CAD build for the part. Positions are in the model's coordinates, mm. Face numbers are marked on the shaded views. Give positions to 0.01 mm unless a question says otherwise; leave off trailing zeros. Loops run counter-clockwise (first coordinate to the right, second up) from the corner with the lowest first, then second, coordinate; pieces in that order, holes last.
```python
from build123d import *

# Parameters (mm, degrees)
BASPROSKE_W         = 8
BASPROSKE_H         = 8.5
TOOTHCUT_DEPTH      = 15.439529078
TEETHCUTS_COUNT     = 15
TEETHCUTS_ANGLE     = 336
BORSKE_R            = 0.75
BORE_DEPTH          = 50.0000508
SKETCH1_R           = 2.8
CUT_EXTRUDE2_DEPTH  = 1
BOSS_EXTRUDE2_START = 1.6
SKETCH2_R           = 0.75
BOSS_EXTRUDE2_DEPTH = 1.6


with BuildPart() as part:
    # BasProSke → Base-Revolve (revolve)
    with BuildSketch(Plane(origin=(0, 0, 0), x_dir=(1, 0, 0), z_dir=(0, 1, 0)), mode=Mode.PRIVATE) as base_revolve_sk:
        with Locations((4, 4.25)):
            Rectangle(BASPROSKE_W, BASPROSKE_H)
    revolve(base_revolve_sk.sketch.rotate(Axis((-10, 0, 0), (1, 0, 0)), 180), axis=Axis((-10, 0, 0), (1, 0, 0)))

    # TooCutSke → ToothCut (cut, through all)
    with BuildSketch(Plane(origin=(0, 0, 0), x_dir=(0, 0, -1), z_dir=(1, 0, 0))):
        with BuildLine():
            ThreePointArc((0.619547138, 6.21821215), (0, 6.249), (-0.619547138, 6.21821215))
            ThreePointArc((-0.619547138, 6.21821215), (-0.827197364, 7.394441061), (-1.477319646, 8.396426134))
            ThreePointArc((-1.477319646, 8.396426134), (0, 8.5254), (1.477319646, 8.396426134))
            ThreePointArc((1.477319646, 8.396426134), (0.827197364, 7.394441061), (0.619547138, 6.21821215))
        make_face()
    toothcut = extrude(amount=TOOTHCUT_DEPTH, mode=Mode.SUBTRACT)

    # TeethCuts: ToothCut ×15 about axis
    teethcuts_axis = Axis((-10, 0, 0), (1, 0, 0))
    for i in range(1, TEETHCUTS_COUNT):
        add(toothcut.rotate(teethcuts_axis, i * TEETHCUTS_ANGLE / (TEETHCUTS_COUNT - 1)), mode=Mode.SUBTRACT)

    # BorSke → Bore (cut, symmetric)
    with BuildSketch(Plane(origin=(0, 0, 0), x_dir=(0, 0, -1), z_dir=(1, 0, 0))):
        with Locations(Location((0, 0, 0), (0, 0, 180))):
            Circle(BORSKE_R)
    extrude(amount=BORE_DEPTH, both=True, mode=Mode.SUBTRACT)

    # Sketch1 → Cut-Extrude2 (cut)
    with BuildSketch(Plane(origin=(8, 0, 0), x_dir=(0, 0, -1), z_dir=(1, 0, 0))):
        Circle(SKETCH1_R)
    extrude(amount=-CUT_EXTRUDE2_DEPTH, mode=Mode.SUBTRACT)

    # Sketch2 → Boss-Extrude2 (add)
    with BuildSketch(Plane.ZY.offset(BOSS_EXTRUDE2_START)):
        with BuildLine():
            ThreePointArc((6.248908444, -0.033826967), (7.425583576, 0.045669992), (8.480693328, 0.572573726))
            ThreePointArc((8.480693328, 0.572573726), (8.453436111, 0.888491938), (8.414414603, 1.203173673))
            ThreePointArc((8.414414603, 1.203173673), (7.272812084, 1.499193643), (6.105321779, 1.332308887))
            ThreePointArc((6.105321779, 1.332308887), (5.94315217, 1.931047198), (5.722420591, 2.510757571))
            ThreePointArc((5.722420591, 2.510757571), (6.765032487, 3.061978551), (7.514612153, 3.972480862))
            ThreePointArc((7.514612153, 3.972480862), (7.361215932, 4.25), (7.197575419, 4.521604593))
            ThreePointArc((7.197575419, 4.521604593), (6.034267454, 4.327700716), (5.035590135, 3.700382817))
            ThreePointArc((5.035590135, 3.700382817), (4.643912014, 4.181397159), (4.206474231, 4.621209316))
            ThreePointArc((4.206474231, 4.621209316), (4.934745822, 5.5488432), (5.249186267, 6.685509968))
            ThreePointArc((5.249186267, 6.685509968), (4.996174644, 6.876644452), (4.736210056, 7.058209001))
            ThreePointArc((4.736210056, 7.058209001), (3.752343161, 6.407909019), (3.095159209, 5.428626941))
            ThreePointArc((3.095159209, 5.428626941), (2.541697283, 5.708745565), (1.963190262, 5.932611987))
            ThreePointArc((1.963190262, 5.932611987), (2.251196774, 7.076262451), (2.076128389, 8.242553664))
            ThreePointArc((2.076128389, 8.242553664), (1.767249372, 8.314254606), (1.455910948, 8.374384951))
            ThreePointArc((1.455910948, 8.374384951), (0.821604647, 7.380131638), (0.619547138, 6.21821215))
            ThreePointArc((0.619547138, 6.21821215), (0, 6.249), (-0.619547138, 6.21821215))
            ThreePointArc((-0.619547138, 6.21821215), (-0.821604647, 7.380131638), (-1.455910948, 8.374384951))
            ThreePointArc((-1.455910948, 8.374384951), (-1.767249372, 8.314254606), (-2.076128389, 8.242553664))
            ThreePointArc((-2.076128389, 8.242553664), (-2.251196774, 7.076262451), (-1.963190262, 5.932611987))
            ThreePointArc((-1.963190262, 5.932611987), (-2.541697283, 5.708745565), (-3.095159209, 5.428626941))
            ThreePointArc((-3.095159209, 5.428626941), (-3.752343161, 6.407909019), (-4.736210056, 7.058209001))
            ThreePointArc((-4.736210056, 7.058209001), (-4.996174644, 6.876644452), (-5.249186267, 6.685509968))
            ThreePointArc((-5.249186267, 6.685509968), (-4.934745822, 5.5488432), (-4.206474231, 4.621209316))
            ThreePointArc((-4.206474231, 4.621209316), (-4.643912014, 4.181397159), (-5.035590135, 3.700382817))
            ThreePointArc((-5.035590135, 3.700382817), (-6.034267454, 4.327700716), (-7.197575419, 4.521604593))
            ThreePointArc((-7.197575419, 4.521604593), (-7.361215932, 4.25), (-7.514612153, 3.972480862))
            ThreePointArc((-7.514612153, 3.972480862), (-6.765032487, 3.061978551), (-5.722420591, 2.510757571))
            ThreePointArc((-5.722420591, 2.510757571), (-5.94315217, 1.931047198), (-6.105321779, 1.332308887))
            ThreePointArc((-6.105321779, 1.332308887), (-7.272812084, 1.499193643), (-8.414414603, 1.203173673))
            ThreePointArc((-8.414414603, 1.203173673), (-8.453436111, 0.888491938), (-8.480693328, 0.572573726))
            ThreePointArc((-8.480693328, 0.572573726), (-7.425583576, 0.045669992), (-6.248908444, -0.033826967))
            ThreePointArc((-6.248908444, -0.033826967), (-6.214767324, -0.653198367), (-6.119387823, -1.266133354))
            ThreePointArc((-6.119387823, -1.266133354), (-7.253821434, -1.58853763), (-8.17632506, -2.323296905))
            ThreePointArc((-8.17632506, -2.323296905), (-8.083980389, -2.626644452), (-7.980385583, -2.926336609))
            ThreePointArc((-7.980385583, -2.926336609), (-6.802183806, -2.978535323), (-5.694903257, -2.572562515))
            ThreePointArc((-5.694903257, -2.572562515), (-5.411792748, -3.1245), (-5.075356119, -3.645649635))
            ThreePointArc((-5.075356119, -3.645649635), (-5.980579158, -4.401596316), (-6.524474635, -5.448048342))
            ThreePointArc((-6.524474635, -5.448048342), (-6.316731017, -5.687610154), (-6.100196671, -5.919256759))
            ThreePointArc((-6.100196671, -5.919256759), (-5.002624659, -5.487724821), (-4.156197561, -4.666478633))
            ThreePointArc((-4.156197561, -4.666478633), (-3.673070042, -5.055547198), (-3.153749234, -5.394799975))
            ThreePointArc((-3.153749234, -5.394799975), (-3.673240415, -6.453579011), (-3.744483272, -7.630782727))
            ThreePointArc((-3.744483272, -7.630782727), (-3.457261466, -7.76513639), (-3.165228336, -7.888683641))
            ThreePointArc((-3.165228336, -7.888683641), (-2.338066262, -7.048036844), (-1.898847548, -5.953518203))
            ThreePointArc((-1.898847548, -5.953518203), (-1.299240156, -6.112444357), (-0.686830456, -6.211140388))
            ThreePointArc((-0.686830456, -6.211140388), (-0.730765033, -7.389679266), (-0.317036734, -8.494085455))
            ThreePointArc((-0.317036734, -8.494085455), (0, -8.5), (0.317036734, -8.494085455))
            ThreePointArc((0.317036734, -8.494085455), (0.730765033, -7.389679266), (0.686830456, -6.211140388))
            ThreePointArc((0.686830456, -6.211140388), (1.299240156, -6.112444357), (1.898847548, -5.953518203))
            ThreePointArc((1.898847548, -5.953518203), (2.338066262, -7.048036844), (3.165228336, -7.888683641))
            ThreePointArc((3.165228336, -7.888683641), (3.457261466, -7.76513639), (3.744483272, -7.630782727))
            ThreePointArc((3.744483272, -7.630782727), (3.673240415, -6.453579011), (3.153749234, -5.394799975))
            ThreePointArc((3.153749234, -5.394799975), (3.673070042, -5.055547198), (4.156197561, -4.666478633))
            ThreePointArc((4.156197561, -4.666478633), (5.002624659, -5.487724821), (6.100196671, -5.919256759))
            ThreePointArc((6.100196671, -5.919256759), (6.316731017, -5.687610154), (6.524474635, -5.448048342))
            ThreePointArc((6.524474635, -5.448048342), (5.980579158, -4.401596316), (5.075356119, -3.645649635))
            ThreePointArc((5.075356119, -3.645649635), (5.411792748, -3.1245), (5.694903257, -2.572562515))
            ThreePointArc((5.694903257, -2.572562515), (6.802183806, -2.978535323), (7.980385583, -2.926336609))
            ThreePointArc((7.980385583, -2.926336609), (8.083980389, -2.626644452), (8.17632506, -2.323296905))
            ThreePointArc((8.17632506, -2.323296905), (7.253821434, -1.58853763), (6.119387823, -1.266133354))
            ThreePointArc((6.119387823, -1.266133354), (6.214767324, -0.653198367), (6.248908444, -0.033826967))
        make_face()
        Circle(SKETCH2_R, mode=Mode.SUBTRACT)
    extrude(amount=-BOSS_EXTRUDE2_DEPTH)


solid = part.part
```
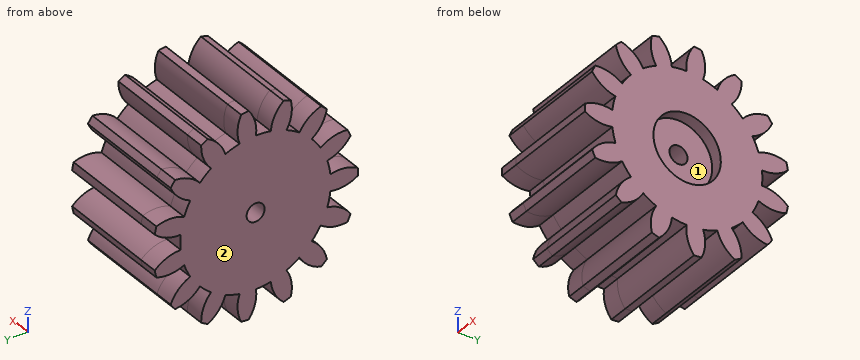
1. Probe line 1 along Y through (x, z) = (7.85, 0); line 2 along Z through (x, y) = (2, 7); line 3 along Z through (x, y) = (1, -7.25). List the from-to ranges inside material, lowest first.
Responses:
line 1: y = -8.5 to -2.8, 2.8 to 6.25
line 2: z = -4.82 to -4.6, -2.25 to -0.7, 0.7 to 2.25, 4.6 to 4.82
line 3: z = -3.77 to -2.48, -0.75 to 0.75, 2.48 to 3.77
2. Drop flat-ended pins along their axis: pin 1 (1.5 mm diameter, centred on x = 5.5, y = -3.5, fed in from -Z); pin 2 (3 mm diameter, centred on x = 1, y = -6.5, fed in from -Z); pin 3 (1 mm diameter, centred on x = 3.5, y = -3, fed in from +Z). Give the stop position or say it passes through.
Responses:
pin 1: stops at z = -8.04
pin 2: stops at z = -6.52
pin 3: stops at z = 8.12
3. Pull direction Z, two halves, no side cores. Call the marked faces 1 and 2: released by +Z, released by -Z, zero draft, split by the parting line, or undercut.
Responses:
face 1: undercut
face 2: zero draft
4. Saw through at A-A, the plane z = 0. List the corners of the cut face in (x, y).
Responses:
outline: (-1.6, -8.5) - (8, -8.5) - (8, -2.8) - (7, -2.8) - (7, -0.75) - (-1.6, -0.75) - close; (-1.6, 0.75) - (7, 0.75) - (7, 2.8) - (8, 2.8) - (8, 6.25) - (-1.6, 6.25) - close
5. Saw through at B-B, the plane y = -7. List the corners of the cut face in (x, z), and give its area (3 significant figures).
Responses:
outline: (-1.6, -3.76) - (8, -3.76) - (8, -2.31) - (-1.6, -2.31) - close; (-1.6, -0.77) - (8, -0.77) - (8, 0.77) - (-1.6, 0.77) - close; (-1.6, 2.31) - (8, 2.31) - (8, 3.76) - (-1.6, 3.76) - close
area: 42.7 mm2
